For this review, take the finished solid that the model builds, in its own axes (mm). Face numbers are marked on the shaded views. A direction names the side the tool comes from. Give positions to 0.01 mm unless a question says otherwise; leave off trailing zeros. Loops run counter-clockwise (first coordinate to the right, second up) from the corner with the lowest first, then second, coordinate; pieces in that order, holes last.
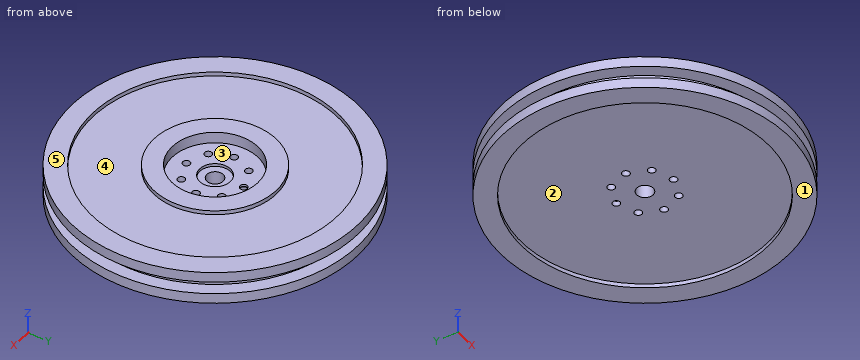
```python
from build123d import *
from build123d.topology import SkipClean

# Parameters (mm, degrees)
SKETCH4_R              = 10.5
CUT_EXTRUDE2_DEPTH     = 2.75
SKETCH5_R              = 3.75
CUT_EXTRUDE3_DEPTH     = 0.7
SKETCH6_R              = 0.9
CUT_EXTRUDE4_DEPTH     = 50.775119287
SKETCH11_R             = 2
CUT_EXTRUDE8_DEPTH     = 50.70616159
CUT_EXTRUDE9_START     = -25
CUT_EXTRUDE9_OUTLINE_R = 1
CUT_EXTRUDE9_DEPTH     = 26
SKETCH18_R             = 30
CUT_EXTRUDE12_DEPTH    = 1
CUT_EXTRUDE13_START    = -1
SKETCH19_R             = 30
SKETCH19_R_2           = 15
CUT_EXTRUDE13_DEPTH    = 1


with BuildPart() as part:
    # Sketch2 → Revolve1 (revolve)
    with BuildSketch(Plane(origin=(0, 0, 0), x_dir=(1, 0, 0), z_dir=(0, 1, 0))):
        Polygon((0, 0), (35, 0), (35, 2.5), (32, 2.5), (32, 5.5), (35, 5.5), (35, 8), (0, 8), align=None)
    revolve(axis=Axis((0, 0, 27.772111005), (0, 0, -1)))

    # Sketch4 → Cut-Extrude2 (cut)
    with BuildSketch(Plane.XY):
        Circle(SKETCH4_R)
    extrude(amount=-CUT_EXTRUDE2_DEPTH, mode=Mode.SUBTRACT)

    # Sketch5 → Cut-Extrude3 (cut)
    with BuildSketch(Plane.XY.offset(-2.75)):
        Circle(SKETCH5_R)
    extrude(amount=-CUT_EXTRUDE3_DEPTH, mode=Mode.SUBTRACT)

    # Sketch6 → Cut-Extrude4 (cut, through all)
    with BuildSketch(Plane.XY.offset(-2.75)):
        with Locations((0, 7)):
            Circle(SKETCH6_R)
        with Locations((4.949747468, 4.949747468)):
            Circle(SKETCH6_R)
        with Locations((7, 0)):
            Circle(SKETCH6_R)
        with Locations((4.949747468, -4.949747468)):
            Circle(SKETCH6_R)
        with Locations((0, -7)):
            Circle(SKETCH6_R)
        with Locations((-4.949747468, -4.949747468)):
            Circle(SKETCH6_R)
        with Locations((-7, 0)):
            Circle(SKETCH6_R)
        with Locations((-4.949747468, 4.949747468)):
            Circle(SKETCH6_R)
    extrude(amount=-CUT_EXTRUDE4_DEPTH, mode=Mode.SUBTRACT)

    # Sketch11 → Cut-Extrude8 (cut, through all)
    with BuildSketch(Plane.XY.offset(-3.45)):
        Circle(SKETCH11_R)
    extrude(amount=-CUT_EXTRUDE8_DEPTH, mode=Mode.SUBTRACT)

    # Cut-Extrude9: read off the stored shape, not the designer's step
    # Cut-Extrude9 outline → Cut-Extrude9 (cut)
    with BuildSketch(Plane(origin=(0, 32, 0), x_dir=(1, 0, 0), z_dir=(0, 1, 0)).offset(CUT_EXTRUDE9_START)):
        with Locations((0, 4.5)):
            Circle(CUT_EXTRUDE9_OUTLINE_R)
    extrude(amount=CUT_EXTRUDE9_DEPTH, mode=Mode.SUBTRACT)

    # Fillet4: read off the stored shape, not the designer's step
    # Fillet4 outline → Fillet4 (revolve, cut)
    with SkipClean():  # the faces are left unmerged after this step: merging them gives an invalid solid
        with BuildSketch(Plane.XZ.offset(-7)):
            with BuildLine():
                Line((1, -5.5), (1, -3.5))
                ThreePointArc((1, -3.5), (0.926138721, -3.398867689), (0.9, -3.276393202))
                Line((0.9, -3.276393202), (0.9, -5.723606798))
                ThreePointArc((0.9, -5.723606798), (0.926138721, -5.601132311), (1, -5.5))
            make_face()
        revolve(axis=Axis((0, 7, 0), (0, 0, 1)), mode=Mode.SUBTRACT)

    # Sketch18 → Cut-Extrude12 (cut)
    with SkipClean():  # the faces are left unmerged after this step: merging them gives an invalid solid
        with BuildSketch(Plane(origin=(0, 0, -8), x_dir=(-1, 0, 0), z_dir=(0, 0, -1))):
            Circle(SKETCH18_R)
        extrude(amount=-CUT_EXTRUDE12_DEPTH, mode=Mode.SUBTRACT)

    # Sketch19 → Cut-Extrude13 (cut)
    with SkipClean():  # the faces are left unmerged after this step: merging them gives an invalid solid
        with BuildSketch(Plane.XY.offset(CUT_EXTRUDE13_START)):
            with Locations(Location((0, 0, 0), (0, 0, 180))):
                Circle(SKETCH19_R)
            Circle(SKETCH19_R_2, mode=Mode.SUBTRACT)
        extrude(amount=CUT_EXTRUDE13_DEPTH, mode=Mode.SUBTRACT)


solid = part.part
```
Q1. Consider section D-D on x = -18.5. Give the boundary of the cut face in (y, z), plus the area to 3 significant figures.
Answers:
outline: (-29.71, -8) - (-23.62, -8) - (-23.62, -7) - (23.62, -7) - (23.62, -8) - (29.71, -8) - (29.71, -5.5) - (26.11, -5.5) - (26.11, -2.5) - (29.71, -2.5) - (29.71, 0) - (23.62, 0) - (23.62, -1) - (-23.62, -1) - (-23.62, 0) - (-29.71, 0) - (-29.71, -2.5) - (-26.11, -2.5) - (-26.11, -5.5) - (-29.71, -5.5) - close
area: 359 mm2
Q2. Mouldability with a two-part tool opening along X and no side actions: class the marked faces 3, 4 and 5 as +X half, -X half, draft (parallel to the pull), parting line (faces both ways), or undercut.
Answers:
face 3: undercut
face 4: undercut
face 5: draft
Q3. Consider section A-A on y = 14. Give the boundary of the cut face in (x, z), plus the area to 3 significant figures.
Answers:
outline: (-32.08, -8) - (-26.53, -8) - (-26.53, -7) - (26.53, -7) - (26.53, -8) - (32.08, -8) - (32.08, -5.5) - (28.77, -5.5) - (28.77, -2.5) - (32.08, -2.5) - (32.08, 0) - (26.53, 0) - (26.53, -1) - (5.39, -1) - (5.39, 0) - (-5.39, 0) - (-5.39, -1) - (-26.53, -1) - (-26.53, 0) - (-32.08, 0) - (-32.08, -2.5) - (-28.77, -2.5) - (-28.77, -5.5) - (-32.08, -5.5) - close; hole circle Ø2 at (0, -4.5)
area: 395 mm2
Q4. Machinability: for the marked faces 1 and 2, which of the approach directions +Z, -Z, +X, -X, +Y, -Y give a long, thin tool a straight path to every point of the face, cutting with its end or side? Answer none if there is none.
Answers:
face 1: -Z, +X, -X, +Y, -Y
face 2: -Z
Q5. For probe 1 along Y at (x, z) = (0, -3); probe 2 along Y at (x, z) = (0, -0.85); probe 3 along Y at (x, z) = (0, -2), list the stretches that pass through material, from the lowest coordinate up.
Answers:
probe 1: y = -32 to -7.9, -6.1 to -3.75, 3.75 to 6.1, 7.9 to 32
probe 2: y = -35 to -30, -15 to -10.5, 10.5 to 15, 30 to 35
probe 3: y = -35 to -10.5, 10.5 to 35
Q6. For pin 1 Ø1 at (y, z) = (27, -2) entering from -X; pin 2 Ø10 at (x, y) = (0, 0) entering from -Z; pin 3 Ø3 at (x, y) = (-4.95, 4.95) entering from +Z; pin 4 Ø1.1 at (x, y) = (0, -7) entering from -Z (3 decimals), all flat-tipped, find the tip position at first contact; note any pin that passes through.
Answers:
pin 1: stops at x = -22.86
pin 2: stops at z = -7
pin 3: stops at z = -2.75
pin 4: passes through
